```python
from build123d import *

# Parameters (mm, degrees)
SKETCH1_W           = 25.4
SKETCH1_H           = 38.1
BOSS_EXTRUDE1_DEPTH = 3.175
SKETCH2_R           = 9.525
SKETCH2_R_2         = 1.778
CUT_EXTRUDE1_DEPTH  = 3.175
SKETCH3_W           = 38.1
SKETCH3_H           = 3.175
BOSS_EXTRUDE2_DEPTH = 38.1
SKETCH6_W           = 38.1
SKETCH6_H           = 3.175
BOSS_EXTRUDE4_DEPTH = 38.1
SKETCH4_R           = 3.175
CUT_EXTRUDE2_DEPTH  = 4.175


with BuildPart() as part:
    # Sketch1 → Boss-Extrude1 (new body)
    with BuildSketch(Plane(origin=(0, 0, 0), x_dir=(1, 0, 0), z_dir=(0, 1, 0))):
        Rectangle(SKETCH1_W, SKETCH1_H)
    extrude(amount=BOSS_EXTRUDE1_DEPTH)

    # Sketch2 → Cut-Extrude1 (cut)
    with BuildSketch(Plane(origin=(0, 3.175, 0), x_dir=(1, 0, 0), z_dir=(0, 1, 0))):
        Circle(SKETCH2_R)
        with Locations((0, -14.5)):
            Circle(SKETCH2_R_2)
        with Locations((0, 14.5)):
            Circle(SKETCH2_R_2)
    extrude(amount=-CUT_EXTRUDE1_DEPTH, mode=Mode.SUBTRACT)

    # Sketch3 → Boss-Extrude2 (add)
    with BuildSketch(Plane.ZY.offset(12.7)):
        with Locations((0, 1.5875)):
            Rectangle(SKETCH3_W, SKETCH3_H)
    extrude(amount=BOSS_EXTRUDE2_DEPTH)

    # Sketch6 → Boss-Extrude4 (add)
    with BuildSketch(Plane(origin=(12.7, 0, 0), x_dir=(0, 0, -1), z_dir=(1, 0, 0))):
        with Locations((0, 1.5875)):
            Rectangle(SKETCH6_W, SKETCH6_H)
    extrude(amount=BOSS_EXTRUDE4_DEPTH)

    # Sketch4 → Cut-Extrude2 (cut, through all)
    with BuildSketch(Plane(origin=(0, 3.175, 0), x_dir=(1, 0, 0), z_dir=(0, 1, 0))):
        with Locations((-44.45, 12.7)):
            Circle(SKETCH4_R)
        with Locations((-44.45, -12.7)):
            Circle(SKETCH4_R)
        with Locations((44.45, -12.7)):
            Circle(SKETCH4_R)
        with Locations((44.45, 12.7)):
            Circle(SKETCH4_R)
    extrude(amount=-CUT_EXTRUDE2_DEPTH, mode=Mode.SUBTRACT)


solid = part.part
```
Read the model definition and answer for the solid it produces. Units are mm, in the model's axes. Give positions to 0.01 mm unless a question says otherwise; leave off trailing zeros. Order: outer loops, then holes, each group sorted by start corner. A loop starts at its lowest first (then second) coordinate and runs counter-clockwise, first axis right, second up. Notation, with made-up numbers: (-12.75, 51) -> (-1.75, 51) arc R22 ccw to (-1.75, 83) -> close; hole circle Ø10 at (63.5, 77.5). An arc over 180 degrees is marked (long way). Write item = value, one per line.
1. A cutting plane is placed at C-C, the plane z = -14.5. Write down the section's boundary in (x, y) (3 decimals).
Numbers:
outline = (-50.8, 0) -> (-47.065, 0) -> (-47.065, 3.175) -> (-50.8, 3.175) -> close; (-41.835, 0) -> (-1.778, 0) -> (-1.778, 3.175) -> (-41.835, 3.175) -> close; (1.778, 0) -> (41.835, 0) -> (41.835, 3.175) -> (1.778, 3.175) -> close; (47.065, 0) -> (50.8, 0) -> (50.8, 3.175) -> (47.065, 3.175) -> close
2. A cutting plane is placed at D-D, the plane z = -2.5. Write down the section's boundary in (x, y) (3 decimals).
Numbers:
outline = (-50.8, 0) -> (-9.191, 0) -> (-9.191, 3.175) -> (-50.8, 3.175) -> close; (9.191, 0) -> (50.8, 0) -> (50.8, 3.175) -> (9.191, 3.175) -> close
3. Straight lines are drawn through the part: line 1 along Z through (x, y) = (-44.45, 1.05) (3 decimals); line 2 along Z through (x, y) = (0, 1.35) (3 decimals); line 3 along X through (y, z) = (1.7, 0) (3 decimals). For each, find the intervals that lie inside material, in ascending order.
Numbers:
line_1 = -19.05 to -15.875, -9.525 to 9.525, 15.875 to 19.05
line_2 = -19.05 to -16.278, -12.722 to -9.525, 9.525 to 12.722, 16.278 to 19.05
line_3 = -50.8 to -9.525, 9.525 to 50.8
4. A cutting plane is placed at A-A, the plane x = 0. Write down the section's boundary in (y, z) (3 decimals), and give its area (3 significant figures).
Numbers:
outline = (0, -19.05) -> (3.175, -19.05) -> (3.175, -16.278) -> (0, -16.278) -> close; (0, -12.722) -> (3.175, -12.722) -> (3.175, -9.525) -> (0, -9.525) -> close; (0, 9.525) -> (3.175, 9.525) -> (3.175, 12.722) -> (0, 12.722) -> close; (0, 16.278) -> (3.175, 16.278) -> (3.175, 19.05) -> (0, 19.05) -> close
area = 37.9 mm²
5. Given pin 1 (5 mm diameter, centred on x = -44.45, z = 12.7, fed in from +Y), flat-ended and moving along its own axis, determine where the tip first touches the part or whether it passes through.
Numbers:
pin_1 = through
6. A cutting plane is placed at B-B, the plane y = 0.9. Write down the section's boundary in (x, z) (3 decimals), and give its area (3 significant figures).
Numbers:
outline = (-50.8, -19.05) -> (50.8, -19.05) -> (50.8, 19.05) -> (-50.8, 19.05) -> close; hole circle Ø6.35 at (-44.45, -12.7); hole circle Ø6.35 at (-44.45, 12.7); hole circle Ø19.05 at (0, 0); hole circle Ø3.556 at (0, -14.5); hole circle Ø3.556 at (0, 14.5); hole circle Ø6.35 at (44.45, -12.7); hole circle Ø6.35 at (44.45, 12.7)
area = 3,440 mm²
7. The mould has two halves that part along Z. Classify faces 1 (the face through (-41.52, 1.61, -11.48)), 2 (the face through (-1, 2, -19.05)), 3 (the face through (-1, 2, 19.05)), 4 (the face through (11, 3.175, 0)): +Z half, -Z half, draft (parallel to the pull), parting line (faces both ways), or undercut.
Numbers:
face_1 = undercut
face_2 = -Z half
face_3 = +Z half
face_4 = draft
